Part model, mm, in its own coordinate system. Face numbers are marked on the shaded views. A direction names the side the tool comes from. Give positions to 0.01 mm unless a question says otherwise; leave off trailing zeros. Write each loop counter-clockwise with the first axis right and the second up, starting at its lowest first coordinate (ties: lowest second). Pieces come first, ordered by that corner, then holes. Notation, with made-up numbers: M 16,31 L 39,31 A32 ccw 39,70 Z; hole C 68.25,33.25 d2. An arc over 180 degrees is marked long. Answer as CSV lines item,"result". Start each with the question number.
Item 1: 3-axis set-ups, long thin cutter, end or side, ignore diameter. For the marked faces 1 and 2: which of +Z, -Z, +X, -X, +Y, -Y reach the whole face in a straight line?
Item 2: Band-saw the part on A-A, the plane x = 6. List the corners of the cut face in (y, z).
Item 3: Wall check: L1, parallel to X at y = -2, z = 2.75; L2, parallel to Y at x = -6, z = -2.5; L3, parallel to X at y = -2.25, z = -1.75. Give the ranges that are in metal, low to high. Write a range as from..to.
Item 4: Pin check, flat tips, straight feed: pin 1 (5 mm diameter, centred on x = 4.5, y = -3.5, fed in from -Z); pin 2 (3 mm diameter, centred on x = 4, z = -3, fed in from -Y); pin 3 (3 mm diameter, centred on x = 0.5, z = 2, fed in from +Y). Stop position of each tip, or through.
from build123d import *

# Parameters (mm, degrees)
SKETCH2_R           = 3
BOSS_EXTRUDE1_DEPTH = 10
CHAMFER1_SIZE       = 0.75
BOSS_EXTRUDE2_DEPTH = 4
SKETCH6_OUTSIDE_W   = 68.106
SKETCH6_OUTSIDE_H   = 69.654
SKETCH6_OUTSIDE_R   = 5
CUT_EXTRUDE1_DEPTH  = 15
CUT_EXTRUDE1_TAPER  = 60


with BuildPart() as part:
    # Sketch2 → Boss-Extrude1 (new body)
    with BuildSketch(Plane(origin=(7, 0, 0), x_dir=(0, 0, -1), z_dir=(1, 0, 0))):
        Circle(SKETCH2_R)
    extrude(amount=-BOSS_EXTRUDE1_DEPTH)

    # Chamfer1
    chamfer1_edges = [part.edges().sort_by_distance(p)[0] for p in [
        (7, 0, 3),
    ]]
    chamfer(chamfer1_edges, length=CHAMFER1_SIZE)

    # Sketch3 → Boss-Extrude2 (add)
    with BuildSketch(Plane.ZY.offset(3)):
        Polygon((-5, -2.886751346), (0, -5.773502692), (5, -2.886751346), (5, 2.886751346), (0, 5.773502692), (-5, 2.886751346), align=None)
    extrude(amount=BOSS_EXTRUDE2_DEPTH)

    # Sketch6 outside → Cut-Extrude1 (cut, through all)
    with BuildSketch(Plane.ZY.offset(7)):
        Rectangle(SKETCH6_OUTSIDE_W, SKETCH6_OUTSIDE_H)
        Circle(SKETCH6_OUTSIDE_R, mode=Mode.SUBTRACT)
    extrude(amount=-CUT_EXTRUDE1_DEPTH, taper=CUT_EXTRUDE1_TAPER, mode=Mode.SUBTRACT)


solid = part.part
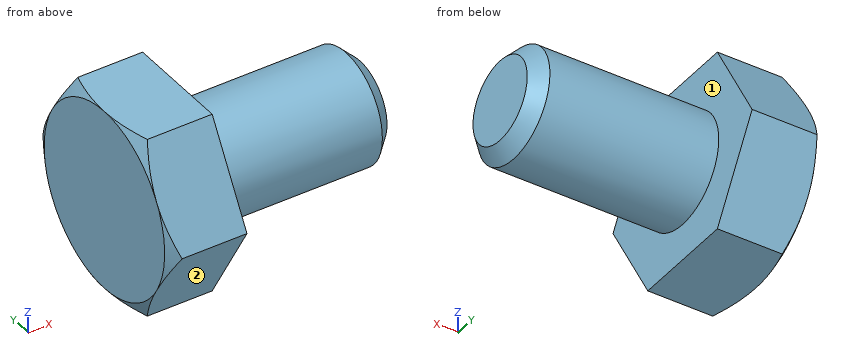
Output:
1,face 1,"+X"
1,face 2,"-Z, +X, -X, -Y"
2,outline,"C 0,0 d6"
3,L1,"-7..-3"
3,L2,"-4.33..4.33"
3,L3,"-7..6.4"
4,pin 1,"z = -2.83"
4,pin 2,"y = -2.6"
4,pin 3,"y = 2.96"
